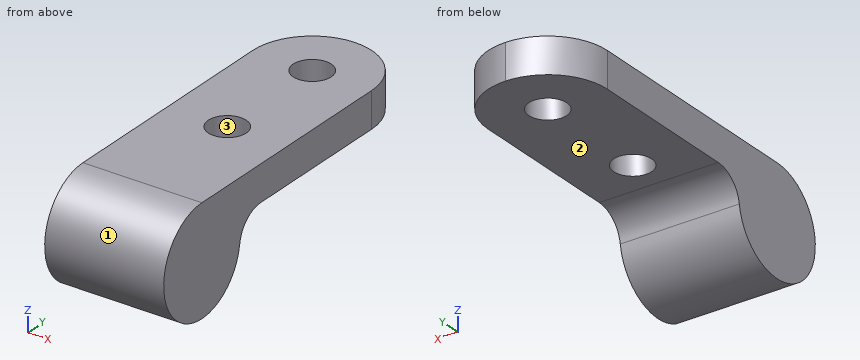
from build123d import *

# Parameters (mm, degrees)
EXTRUDE_1_DEPTH     = 10
SKETCH_3_R          = 1.6
CUT_EXTRUDE_1_DEPTH = 28.586228448


with BuildPart() as part:
    # 草图2 → 凸台-拉伸1 (new body)
    with BuildSketch(Plane(origin=(0, 0, 0), x_dir=(0, 0, -1), z_dir=(1, 0, 0))):
        with BuildLine():
            Line((-4.5, 25), (-1.5, 25))
            Line((-1.5, 25), (-1.5, 6.92820323))
            ThreePointArc((-1.5, 6.92820323), (-0.889822365, 5.291569054), (0.642857143, 4.453844934))
            ThreePointArc((0.642857143, 4.453844934), (2.945941518, -3.401680257), (-4.5, 0))
            Line((-4.5, 0), (-4.5, 25))
        make_face()
    extrude(amount=EXTRUDE_1_DEPTH)

    # 草图3 → 切除-拉伸1 (cut, through all)
    with BuildSketch(Plane(origin=(0, 0, 1.5), x_dir=(-1, 0, 0), z_dir=(0, 0, -1))):
        with BuildLine():
            Line((-10, 25), (-10, 20))
            ThreePointArc((-10, 20), (-8.535533906, 23.535533906), (-5, 25))
            Line((-5, 25), (-10, 25))
        make_face()
        with BuildLine():
            Line((0, 25), (-5, 25))
            ThreePointArc((-5, 25), (-1.464466094, 23.535533906), (0, 20))
            Line((0, 20), (0, 25))
        make_face()
        with Locations(Location((-5, 20, 0), (0, 0, 90))):
            Circle(SKETCH_3_R)
        with Locations(Location((-5, 10, 0), (0, 0, 90))):
            Circle(SKETCH_3_R)
    extrude(amount=-CUT_EXTRUDE_1_DEPTH, mode=Mode.SUBTRACT)


solid = part.part
Geometry check sheet. Reference: the model listing, model coordinates, mm. Face numbers are marked on the shaded views. Round coordinates to 2 decimals unless told otherwise and drop trailing zeros. Loops run counter-clockwise (first coordinate to the right, second up) from the corner with the lowest first, then second, coordinate; pieces in that order, holes last. Notation, with made-up numbers: (-36.75, 14) - (-12.75, 14) arc R32 ccw to (-12.75, 52) - close; hole circle Ø10 at (2, -23). An arc over 180 degrees is marked (long way). One line per question, with ' | ' between items. Start each with the question number.
1. Scan lines: line 1 (X direction, y = 10, z = 2.75); line 2 (Z direction, x = 4, y = 17.25); line 3 (Y direction, x = 4, z = 3.5). Record each from-to range of solid material in increasing order. Write a range as [from, to].
2. Cross-section at D-D on z = -1.75. Record the cut outline in (x, y), then the cut area to 3 significant figures.
3. Cross-section at C-C on y = 7.25. Record the cut outline in (x, z).
4. Depth check by flat-ended pin: pin 1 (5 mm diameter, centred on x = 6.5, y = 21.5, fed in from -Z); pin 2 (1 mm diameter, centred on x = 3, z = -1, fed in from +Y); pin 3 (3 mm diameter, centred on x = 6, z = 3, fed in from -Y); pin 4 (3 mm diameter, centred on x = 5, y = 10, fed in from -Z). Enter the tip coordinate at first touch or a pass-through.
5. Cross-section at B-B on x = 2. Record the cut outline in (y, z), then the cut area to 3 significant figures.
6. Cross-section at A-A on y = 21.25. Record the cut outline in (x, z).
7. Draft check along Y on the marked faces 1, 2 and 3. Enter one of: released by +Y, released by -Y, zero draft, split by the parting line, or undercut.
Taken from the geometry:
1) line 1: [0, 3.4], [6.6, 10] | line 2: [1.5, 4.5] | line 3: [-2.83, 8.75], [11.25, 18.75], [21.25, 24.9]
2) outline: (0, -4.15) - (10, -4.15) - (10, 4.15) - (0, 4.15) - close | area: 82.9 mm²
3) outline: (0, 1.5) - (10, 1.5) - (10, 4.5) - (0, 4.5) - close
4) pin 1: z = 1.5 | pin 2: y = 4.48 | pin 3: y = -4.24 | pin 4: through
5) outline: (0, 4.5) arc R4.5 ccw (long way) to (4.45, -0.64) arc R2.5 cw to (6.93, 1.5) - (24, 1.5) - (24, 4.5) - close | area: 128 mm²
6) outline: (0.16, 1.5) - (4, 1.5) - (4, 4.5) - (0.16, 4.5) - close; (6, 1.5) - (9.84, 1.5) - (9.84, 4.5) - (6, 4.5) - close
7) face 1: split by the parting line | face 2: zero draft | face 3: undercut
